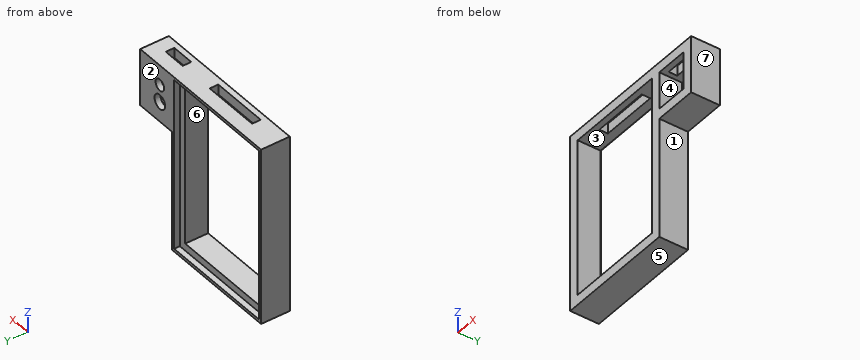
from build123d import *

# Parameters (mm, degrees)
CROQUIS1_W              = 42
CROQUIS1_H              = 62
SALIENTE_EXTRUIR1_DEPTH = 10
CROQUIS2_W              = 40
CROQUIS2_H              = 60
CORTAR_EXTRUIR1_DEPTH   = 2
CROQUIS3_W              = 35
CROQUIS3_H              = 55
CORTAR_EXTRUIR2_DEPTH   = 8
CROQUIS4_W              = 20
CROQUIS4_H              = 3
CORTAR_EXTRUIR3_DEPTH   = 8
CROQUIS5_W              = 20
CROQUIS5_H              = 10
SALIENTE_EXTRUIR2_DEPTH = 15
CROQUIS6_W              = 11.5
CROQUIS6_H              = 13
CORTAR_EXTRUIR4_DEPTH   = 8
CROQUIS7_R              = 2.5
CROQUIS7_R_2            = 2
CORTAR_EXTRUIR5_DEPTH   = 8
CROQUIS8_W              = 8
CROQUIS8_H              = 3
CORTAR_EXTRUIR6_DEPTH   = 8


with BuildPart() as part:
    # Croquis1 → Saliente-Extruir1 (new body)
    with BuildSketch(Plane(origin=(0, 0, 0), x_dir=(1, 0, 0), z_dir=(0, 1, 0))):
        Rectangle(CROQUIS1_W, CROQUIS1_H)
    extrude(amount=SALIENTE_EXTRUIR1_DEPTH)

    # Croquis2 → Cortar-Extruir1 (cut)
    with BuildSketch(Plane(origin=(0, 10, 0), x_dir=(1, 0, 0), z_dir=(0, 1, 0))):
        Rectangle(CROQUIS2_W, CROQUIS2_H)
    extrude(amount=-CORTAR_EXTRUIR1_DEPTH, mode=Mode.SUBTRACT)

    # Croquis3 → Cortar-Extruir2 (cut)
    with BuildSketch(Plane(origin=(0, 8, 0), x_dir=(1, 0, 0), z_dir=(0, 1, 0))):
        Rectangle(CROQUIS3_W, CROQUIS3_H)
    extrude(amount=-CORTAR_EXTRUIR2_DEPTH, mode=Mode.SUBTRACT)

    # Croquis4 → Cortar-Extruir3 (cut)
    with BuildSketch(Plane.XY.offset(31)):
        with Locations((0, 3.5)):
            Rectangle(CROQUIS4_W, CROQUIS4_H)
    extrude(amount=-CORTAR_EXTRUIR3_DEPTH, mode=Mode.SUBTRACT)

    # Croquis5 → Saliente-Extruir2 (add)
    with BuildSketch(Plane(origin=(21, 0, 0), x_dir=(0, 0, -1), z_dir=(1, 0, 0))):
        with Locations((-21, 5)):
            Rectangle(CROQUIS5_W, CROQUIS5_H)
    extrude(amount=SALIENTE_EXTRUIR2_DEPTH)

    # Croquis6 → Cortar-Extruir4 (cut)
    with BuildSketch(Plane(origin=(0, 0, 0), x_dir=(-1, 0, 0), z_dir=(0, -1, 0))):
        with Locations((-26.75, -21)):
            Rectangle(CROQUIS6_W, CROQUIS6_H)
    extrude(amount=-CORTAR_EXTRUIR4_DEPTH, mode=Mode.SUBTRACT)

    # Croquis7 → Cortar-Extruir5 (cut)
    with BuildSketch(Plane(origin=(0, 10, 0), x_dir=(1, 0, 0), z_dir=(0, 1, 0))):
        with Locations((26.75, -18)):
            Circle(CROQUIS7_R)
        with Locations((26.75, -24)):
            Circle(CROQUIS7_R_2)
    extrude(amount=-CORTAR_EXTRUIR5_DEPTH, mode=Mode.SUBTRACT)

    # Croquis8 → Cortar-Extruir6 (cut)
    with BuildSketch(Plane.XY.offset(31)):
        with Locations((26.75, 3.5)):
            Rectangle(CROQUIS8_W, CROQUIS8_H)
    extrude(amount=-CORTAR_EXTRUIR6_DEPTH, mode=Mode.SUBTRACT)


solid = part.part
Source: CAD feature listing. Evaluate the final solid. Frame: model axes, mm. Face numbers are marked on the shaded views. A direction names the side the tool comes from. Give positions to 0.01 mm unless a question says otherwise; leave off trailing zeros. Order: outer loops, then holes, each group sorted by start corner. A loop starts at its lowest first (then second) coordinate and runs counter-clockwise, first axis right, second up. Notation, with made-up numbers: (39.25, 76) -> (78.25, 76) arc R11 cw to (78.25, 90) -> close; hole circle Ø1 at (31, 33.5). An arc over 180 degrees is marked (long way). Use a Markdown table: item, result.
1) Section query C-C, the plane y = 1.25. Return the cut outline in (x, z).
Answer list:
| item | result |
|---|---|
| outline | (-21, -31) -> (21, -31) -> (21, 11) -> (36, 11) -> (36, 31) -> (-21, 31) -> close; hole (-17.5, -27.5) -> (17.5, -27.5) -> (17.5, 27.5) -> (-17.5, 27.5) -> close; hole (21, 14.5) -> (32.5, 14.5) -> (32.5, 27.5) -> (21, 27.5) -> close |
2) Section query B-B, the plane z = 24. Return the cut outline in (x, y), then the cut area to 3 significant figures.
Answer list:
| item | result |
|---|---|
| outline | (-21, 0) -> (-17.5, 0) -> (-17.5, 8) -> (-20, 8) -> (-20, 10) -> (-21, 10) -> close; (17.5, 0) -> (21, 0) -> (21, 8) -> (24.75, 8) -> (24.75, 10) -> (20, 10) -> (20, 8) -> (17.5, 8) -> close; (28.75, 8) -> (32.5, 8) -> (32.5, 0) -> (36, 0) -> (36, 10) -> (28.75, 10) -> close |
| area | 110 mm² |
3) Ray query, line 1 along Z through (x, y) = (26.75, 8.4); line 2 along X through (y, z) = (4.5, -10); line 3 along X through (y, z) = (8.75, 24). Return the intervals inside material, ascending. Write a range as [from, to].
Answer list:
| item | result |
|---|---|
| line 1 | [11, 15.5], [20.5, 22], [26, 31] |
| line 2 | [-21, -17.5], [17.5, 21] |
| line 3 | [-21, -20], [20, 24.75], [28.75, 36] |
4) Mould query, pull axis Z, two halves, no side actions, for the marked faces 5, 6 and 7. Classes: +Z half, -Z half, draft (parallel to the pull), parting line (faces both ways), or undercut.
Answer list:
| item | result |
|---|---|
| face 5 | -Z half |
| face 6 | undercut |
| face 7 | draft |
5) Reachability of the marked faces 1, 2, 3 and 4 from +Z, -Z, +X, -X, +Y, -Y: full face, straight path, thin tool, end or side. Return the list, or none.
Answer list:
| item | result |
|---|---|
| face 1 | -Z, +X, +Y, -Y |
| face 2 | +Z, -Z, +X, -X, +Y |
| face 3 | +Y, -Y |
| face 4 | -Y |
6) Section query A-A, the plane x = -7.5. Return the cut outline in (y, z).
Answer list:
| item | result |
|---|---|
| outline | (0, -31) -> (10, -31) -> (10, -30) -> (8, -30) -> (8, -27.5) -> (0, -27.5) -> close; (0, 27.5) -> (2, 27.5) -> (2, 31) -> (0, 31) -> close; (5, 27.5) -> (8, 27.5) -> (8, 30) -> (10, 30) -> (10, 31) -> (5, 31) -> close |
7) Contact query for a flat-ended pin moving along its axis: P1, Ø12, axis at x = -9.5, z = 14.5, coming from the +Y side. Output: stop coordinate, or through.
Answer list:
| item | result |
|---|---|
| P1 | through |
8) Section query D-D, the plane x = 26.75. Return the cut outline in (y, z).
Answer list:
| item | result |
|---|---|
| outline | (0, 11) -> (10, 11) -> (10, 15.5) -> (8, 15.5) -> (8, 14.5) -> (0, 14.5) -> close; (0, 27.5) -> (2, 27.5) -> (2, 31) -> (0, 31) -> close; (5, 27.5) -> (8, 27.5) -> (8, 26) -> (10, 26) -> (10, 31) -> (5, 31) -> close; (8, 20.5) -> (10, 20.5) -> (10, 22) -> (8, 22) -> close |
